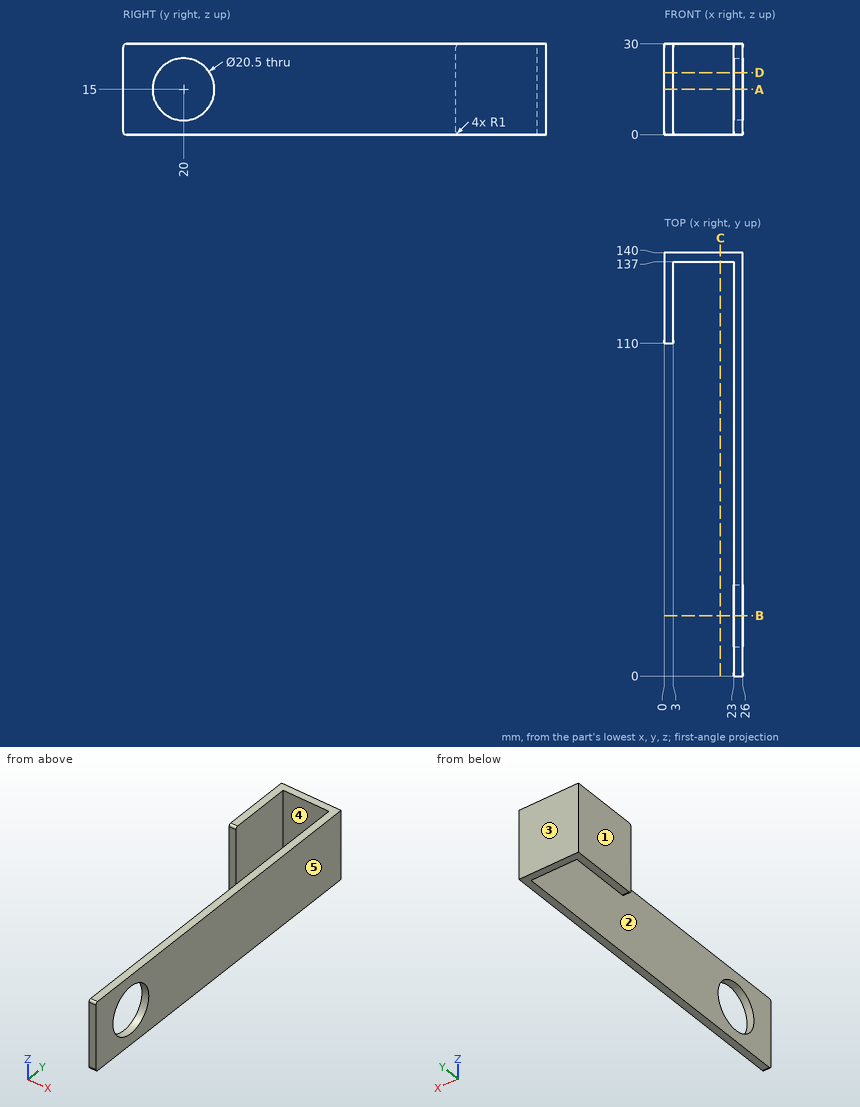
For this review, use the dimensioned drawing (mm, ordinates from the lowest corner) and the shaded views. A direction names the side the tool comes from. Give positions to 0.01 mm unless a question says otherwise; leave off trailing zeros. Order: outer loops, then holes, each group sorted by start corner. A loop starts at its lowest first (then second) coordinate and runs counter-clockwise, first axis right, second up. Notation, with made-up numbers: (77, -11.5) - (119, -11.5) arc R20 cw to (119, 16.5) - close; hole circle Ø4 at (30.5, -12.75). An arc over 180 degrees is marked (long way). Use CSV: the item, a comma, the result in double quotes. Start each with the question number.
Q1. We need section C-C, the plane x = 18.5. Write out the cut boundary in (y, z), and give its area (3 significant figures).
Q2. To check wall thickness, follow line 1 along X through (y, z) = (121, 19.75); line 2 along Y through (x, z) = (24.8, 15); line 3 along X through (y, z) = (30, 11.5). State the ranges of each line that lie inside material, in increasing order. Write a range as [from, to].
Q3. Tool access review of the marked faces 4 and 5: name each direction out of +Z, -Z, +X, -X, +Y, -Y from which nothing blocks a thin tool from reaching the whole face with its end or side.
Q4. Clearance check with flat-ended pins moving along their axes: pin 1 Ø12 at (x, z) = (7, 10) entering from -Y; pin 2 Ø3 at (x, z) = (22.5, 13.5) entering from -Y; pin 3 Ø6 at (y, z) = (61.5, 19.5) entering from -X; pin 4 Ø6 at (x, z) = (11.5, 12.5) entering from -Y. State where each tip first meets the part, or that it passes through.
Q5. The part is to be moulded in two halves that separate along X. For the marked faces 1, 2 and 3, say which applies: +X half, -X half, draft (parallel to the pull), parting line (faces both ways), or undercut.
Q6. We need section B-B, the plane y = 20. Write out the cut boundary in (x, z).
Q7. We need section A-A, the plane z = 15. Write out the cut boundary in (x, y).
Q8. We need section D-D, the plane z = 20.5. Write out the cut boundary in (x, y).
Outcome:
1,outline,"(137, 0) - (140, 0) - (140, 30) - (137, 30) - close"
1,area,"90.0 mm^2"
2,line 1,"x = [0, 3], [23, 26]"
2,line 2,"y = [0, 9.75], [30.25, 140]"
2,line 3,"x = [23, 26]"
3,face 4,"+Z, -Z, -Y"
3,face 5,"+Z, -Z, +X, +Y, -Y"
4,pin 1,"stops at y = 110"
4,pin 2,"stops at y = 0"
4,pin 3,"stops at x = 23"
4,pin 4,"stops at y = 137"
5,face 1,"-X half"
5,face 2,"undercut"
5,face 3,"draft"
6,outline,"(23, 0) - (26, 0) - (26, 4.75) - (23, 4.75) - close; (23, 25.25) - (26, 25.25) - (26, 30) - (23, 30) - close"
7,outline,"(0, 110) - (3, 110) - (3, 137) - (23, 137) - (23, 30.25) - (26, 30.25) - (26, 140) - (0, 140) - close; (23, 0) - (26, 0) - (26, 9.75) - (23, 9.75) - close"
8,outline,"(0, 110) - (3, 110) - (3, 137) - (23, 137) - (23, 28.65) - (26, 28.65) - (26, 140) - (0, 140) - close; (23, 0) - (26, 0) - (26, 11.35) - (23, 11.35) - close"
